from build123d import *

# Parameters (mm, degrees)
ESQUISSE1_W             = 186
ESQUISSE1_H             = 330
BOSS_EXTRU_1_DEPTH      = 6
ESQUISSE3_R             = 2
ESQUISSE3_R_2           = 10
ESQUISSE3_R_3           = 1.4
ESQUISSE3_W             = 55
ESQUISSE3_H             = 8
ESQUISSE3_H_2           = 44
ENL_V_MAT_EXTRU_2_DEPTH = 6
ESQUISSE4_W             = 6
ESQUISSE4_H             = 181
ENL_V_MAT_EXTRU_3_DEPTH = 379.856173237


with BuildPart() as part:
    # Esquisse1 → Boss.-Extru.1 (new body)
    with BuildSketch(Plane.XY):
        with Locations((-93, 165)):
            Rectangle(ESQUISSE1_W, ESQUISSE1_H)
    extrude(amount=BOSS_EXTRU_1_DEPTH)

    # Esquisse3 → Enlèv. mat.-Extru.2 (cut)
    with BuildSketch(Plane.XY.offset(6)):
        with Locations((-4, 4)):
            Circle(ESQUISSE3_R)
        with Locations((-20, 25)):
            Circle(ESQUISSE3_R_2)
        with Locations((-20, 39.73)):
            Circle(ESQUISSE3_R_3)
        with Locations((-20, 54.73)):
            Circle(ESQUISSE3_R_3)
        with Locations(Location((-20, 275.27, 0), (0, 0, 180))):
            Circle(ESQUISSE3_R_3)
        with Locations(Location((-20, 290.27, 0), (0, 0, 180))):
            Circle(ESQUISSE3_R_3)
        with Locations(Location((-4, 326, 0), (0, 0, 180))):
            Circle(ESQUISSE3_R)
        with Locations(Location((-20, 305, 0), (0, 0, 180))):
            Circle(ESQUISSE3_R_2)
        with Locations((-68.25, 11)):
            Rectangle(ESQUISSE3_W, ESQUISSE3_H)
        with Locations((-68.25, 57)):
            Rectangle(ESQUISSE3_W, ESQUISSE3_H_2)
        with Locations((-68.25, 273)):
            Rectangle(ESQUISSE3_W, ESQUISSE3_H_2)
        with Locations((-68.25, 319)):
            Rectangle(ESQUISSE3_W, ESQUISSE3_H)
    extrude(amount=-ENL_V_MAT_EXTRU_2_DEPTH, mode=Mode.SUBTRACT)

    # Esquisse4 → Enlèv. mat.-Extru.3 (cut, through all)
    with BuildSketch(Plane(origin=(0, 0, 0), x_dir=(-1, 0, 0), z_dir=(0, 0, -1))):
        with Locations((183, 165)):
            Rectangle(ESQUISSE4_W, ESQUISSE4_H)
    extrude(amount=-ENL_V_MAT_EXTRU_3_DEPTH, mode=Mode.SUBTRACT)


solid = part.part
The model under review builds one solid part; all positions refer to its coordinate system, in mm. A direction names the side the tool comes from. Round coordinates to 2 decimals unless told otherwise and drop trailing zeros. Write each loop counter-clockwise with the first axis right and the second up, starting at its lowest first coordinate (ties: lowest second). Pieces come first, ordered by that corner, then holes. Notation, with made-up numbers: M 10.25,36 L 22.25,36 A24 ccw 22.25,53 Z; hole C -38.5,-33.5 d10. An arc over 180 degrees is marked long. Answer as CSV lines item,"result". Start each with the question number.
Q1. Consider section C-C, the plane z = 1.25. State how many separate pieces and enclosed holes the cut face has, then the cut area to 3 significant figures.
Q2. Clearance check with a flat-ended pin moving along its axis: P1, Ø1, axis at y = 83.5, z = 3.5, coming from the +X side. State where the tip first meets the part, or that it passes through.
Q3. Consider section D-D, the plane y = 305. Give the boundary of the cut face in (x, z), then the cut area to 3 significant figures.
Q4. Wall thickness on line 1 along X through (y, z) = (290.27, 4.6); line 2 along Y through (x, z) = (-64.5, 1.05); line 3 along X through (y, z) = (326, 4.65): over which ranges is each line inside the solid? List them lowest first.
Q5. Consider section A-A, the plane x = -86.5. Give the boundary of the cut face in (y, z).
Q6. Tool access review of faces 4 (the face through (-183, 74.5, 3)), 5 (the face through (-95.75, 57, 3)), 6 (the face through (-186, 292, 3)): name each direction out of +Z, -Z, +X, -X, +Y, -Y from which nothing blocks a thin tool from reaching the whole face with its end or side.
Q7. Consider section B-B, the plane y = 270. Give the boundary of the cut face in (x, z), then the cut area to 3 significant figures.
Q8. The part is to be moulded in two halves that separate along X. For faces 1 (the face through (0, 163, 3)), 2 (the face through (-40.75, 11, 3)), 3 (the face through (-94, 0, 3)), say which applies: +X half, -X half, draft (parallel to the pull), parting line (faces both ways), or undercut.
Result set:
1,separate pieces,"1"
1,enclosed holes,"12"
1,area,"53,900 mm²"
2,P1,"stops at x = 0"
3,outline,"M -186,0 L -30,0 L -30,6 L -186,6 Z; M -10,0 L 0,0 L 0,6 L -10,6 Z"
3,area,"996 mm²"
4,line 1,"x = -186 to -95.75, -40.75 to -21.4, -18.6 to 0"
4,line 2,"y = 0 to 7, 15 to 35, 79 to 251, 295 to 315, 323 to 330"
4,line 3,"x = -186 to -6, -2 to 0"
5,outline,"M 0,0 L 7,0 L 7,6 L 0,6 Z; M 15,0 L 35,0 L 35,6 L 15,6 Z; M 79,0 L 251,0 L 251,6 L 79,6 Z; M 295,0 L 315,0 L 315,6 L 295,6 Z; M 323,0 L 330,0 L 330,6 L 323,6 Z"
6,face 4,"+Z, -Z, -X"
6,face 5,"+Z, -Z"
6,face 6,"+Z, -Z, -X, +Y, -Y"
7,outline,"M -186,0 L -95.75,0 L -95.75,6 L -186,6 Z; M -40.75,0 L 0,0 L 0,6 L -40.75,6 Z"
7,area,"786 mm²"
8,face 1,"+X half"
8,face 2,"undercut"
8,face 3,"draft"
